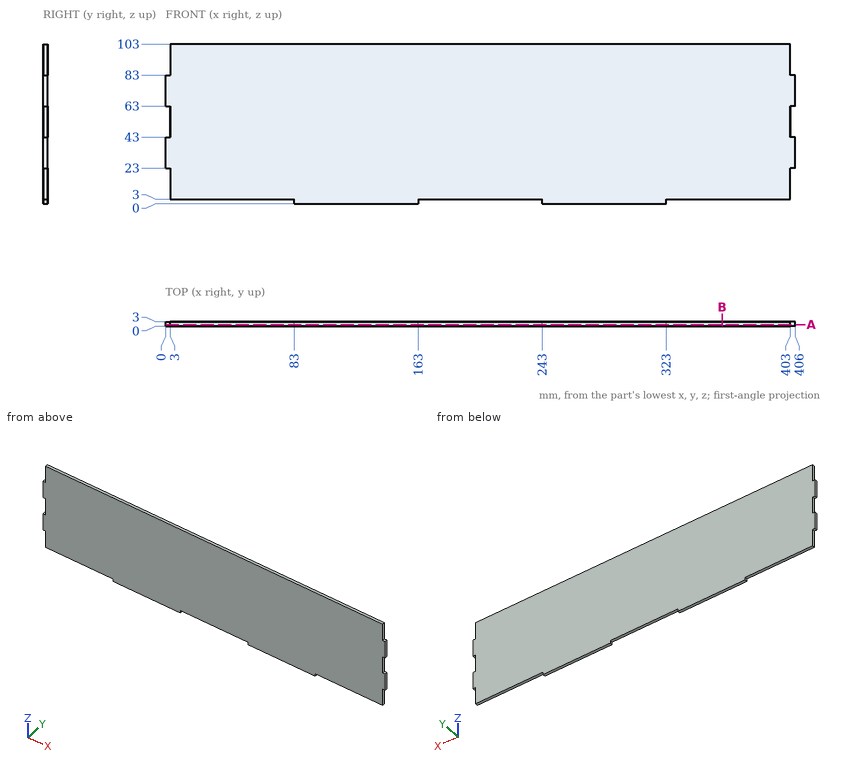
Could you check a few things on this drawing? It's one solid part, dimensions in mm from its lowest x, y, z. Round coordinates to 2 decimals unless told otherwise and drop trailing zeros. Order: outer loops, then holes, each group sorted by start corner. A loop starts at its lowest first (then second) coordinate and runs counter-clockwise, first axis right, second up. Notation, with made-up numbers: M 40.25,49.25 L 45.25,49.25 A4 ccw 45.25,56.25 Z; hole C 66.25,-12.5 d10. An arc over 180 degrees is marked long. Use a Markdown table: item, result.
1) Imagine slicing it at B-B (x = 359). List the corners of the cut face in (y, z) for me, then the cut area to 3 significant figures.
Geometry says:
| item | result |
|---|---|
| outline | M 0,3 L 3,3 L 3,103 L 0,103 Z |
| area | 300 mm² |
2) If I drill on line 1 along X through (y, z) = (2.3, 85); line 2 along Z through (x, y) = (364, 1.45), over which ranges is the centre line in solid material (lowest first)?
Geometry says:
| item | result |
|---|---|
| line 1 | x = 3 to 403 |
| line 2 | z = 3 to 103 |
3) Imagine slicing it at A-A (y = 1.1). List the corners of the cut face in (x, z) for me.
Geometry says:
| item | result |
|---|---|
| outline | M 0,23 L 3,23 L 3,3 L 83,3 L 83,0 L 163,0 L 163,3 L 243,3 L 243,0 L 323,0 L 323,3 L 403,3 L 403,23 L 406,23 L 406,43 L 403,43 L 403,63 L 406,63 L 406,83 L 403,83 L 403,103 L 3,103 L 3,83 L 0,83 L 0,63 L 3,63 L 3,43 L 0,43 Z |
4) I'm going to push flat-ended pins straight in: P1, Ø1.5, axis at x = 404.5, y = 2, coming from the -Z side; P2, Ø0.9, axis at y = 1, z = 1.5, coming from the +X side; P3, Ø0.9, axis at y = 2, z = 91, coming from the +X side. Where does each tip first touch, or does it pass through?
Geometry says:
| item | result |
|---|---|
| P1 | stops at z = 23 |
| P2 | stops at x = 323 |
| P3 | stops at x = 403 |
